Read the model definition and answer for the solid it produces. Units are mm, in the model's axes. Face numbers are marked on the shaded views. A direction names the side the tool comes from. Coordinates: 2 decimals unless noted, no trailing zeros. Loops run counter-clockwise (first coordinate to the right, second up) from the corner with the lowest first, then second, coordinate; pieces in that order, holes last. Notation, with made-up numbers: (7.25, 61.25) - (28.25, 61.25) arc R10 cw to (28.25, 66.25) - close; hole circle Ø5 at (32, 84). An arc over 180 degrees is marked (long way). Use one line per item in the form item = value.
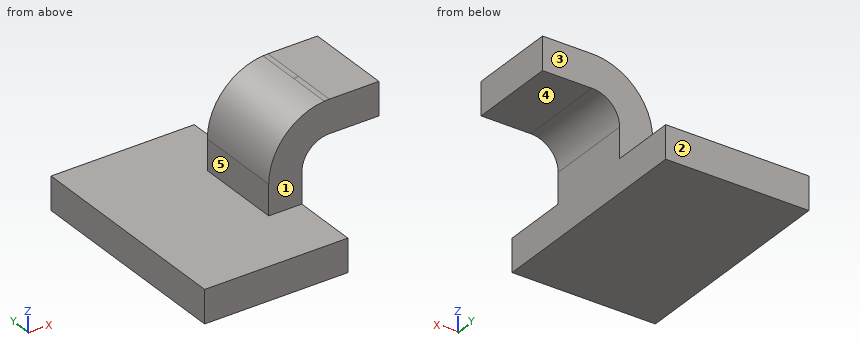
from build123d import *

# Parameters (mm, degrees)
F1_DEPTH = 63.5
F0_W     = 25.4
F0_H     = 19.05
F2_DEPTH = 25.4


with BuildPart() as f1:
    # F0 (on Front) → F1 (new body, symmetric)
    with BuildSketch(Plane.XZ):
        Polygon((-41.275, 9.525), (-41.275, -9.525), (41.275, -9.525), (41.275, 9.525), (22.225, 9.525), align=None)
    extrude(amount=F1_DEPTH, both=True)

    # F0 (on Front) → F2 (join, symmetric)
    with BuildSketch(Plane.XZ):
        with BuildLine():
            Line((22.225, 9.525), (41.275, 9.525))
            Line((41.275, 9.525), (41.275, 27.0002))
            ThreePointArc((41.275, 27.0002), (45.9246798487, 38.2255201513), (57.15, 42.8752))
            Line((57.15, 42.8752), (60.325, 42.8752))
            Line((60.325, 42.8752), (60.325, 61.9252))
            Line((60.325, 61.9252), (57.15, 61.9252))
            add(Edge.make_bspline(
                [(54.2509610844, 61.8046709537), (55.223787741, 61.8579046619), (56.1904041121, 61.8981915291), (57.15, 61.9252)],
                knots=[108.9688631061, 108.9688631061, 108.9688631061, 108.9688631061, 111.5045361635, 111.5045361635, 111.5045361635, 111.5045361635], degree=3))
            ThreePointArc((54.2509610844, 61.8046709537), (31.4497610991, 50.6487379133), (22.225, 27.0002))
            Line((22.225, 27.0002), (22.225, 9.525))
        make_face()
        with Locations((73.025, 52.4002)):
            Rectangle(F0_W, F0_H)
    extrude(amount=F2_DEPTH, both=True)


solid = f1.part
Item 1: Each of these flat-tipped pins is pushed along its axis until it touches: P1, Ø15.5, axis at x = 50, z = 41, coming from the +Y side; P2, Ø2, axis at y = -10.5, z = 15.5, coming from the +X side (3 decimals); P3, Ø14, axis at y = -11.5, z = 17.5, coming from the -X side (3 decimals). Where does it stop, or does it pass through?
Results below:
P1 = 25.4
P2 = 41.275
P3 = 22.225
Item 2: Which of the six approach directions +Z, -Z, +X, -X, +Y, -Y give full straight-line access (tool end or side, diameter ignored) to the marked faces 1, 2, 3, 4 and 5?
Results below:
face_1 = +Z, +X, -X, -Y
face_2 = +Z, -Z, +X, -X, +Y
face_3 = +Z, +X, -X, +Y
face_4 = -Z, +X, +Y, -Y
face_5 = +Z, -X, +Y, -Y
Item 3: The part is cut by section B-B on x = 29. Give the vertices of the cut face in (y, z) (3 decimals).
Results below:
outline = (-63.5, -9.525) - (63.5, -9.525) - (63.5, 9.525) - (25.4, 9.525) - (25.4, 47.672) - (-25.4, 47.672) - (-25.4, 9.525) - (-63.5, 9.525) - close
Item 4: The part is cut by section C-C on y = 44.5. Give the vertices of the cut face in (x, z) (3 decimals).
Results below:
outline = (-41.275, -9.525) - (41.275, -9.525) - (41.275, 9.525) - (-41.275, 9.525) - close
Item 5: Find the intervals of material crossed by L1, parallel to X at y = 23, z = 12.5 (3 decimals); L2, parallel to Z at x = -29, y = 27.5 (3 decimals); L3, parallel to X at y = -1, z = -3 (3 decimals), in increasing order.
Results below:
L1 = 22.225 to 41.275
L2 = -9.525 to 9.525
L3 = -41.275 to 41.275
Item 6: The part is cut by section A-A on z = 7. Give the vertices of the cut face in (x, y) (3 decimals).
Results below:
outline = (-41.275, -63.5) - (41.275, -63.5) - (41.275, 63.5) - (-41.275, 63.5) - close
